from build123d import *

# Parameters (mm, degrees)
F1_DEPTH = 30
F2_R     = 3


with BuildPart() as f1:
    # F0 (on Front) → F1 (new body)
    with BuildSketch(Plane.XZ):
        with BuildLine():
            ThreePointArc((180, -20.182252), (0, -38.788033), (-180, -20.182252))
            Line((-180, -20.182252), (-180, -58.968014))
            ThreePointArc((-180, -58.968014), (0, -76.788032), (180, -58.968014))
            Line((180, -58.968014), (180, -20.182252))
        make_face()
    extrude(amount=-F1_DEPTH)

    # F2
    f2_edges = [f1.edges().sort_by_distance(p)[0] for p in [
        (-180, 15, -20.182252),
        (-180, 15, -58.968014),
        (-180, 0, -39.575133),
        (-180, 30, -39.575133),
        (180, 15, -58.968014),
        (180, 15, -20.182252),
        (180, 0, -39.575133),
        (180, 30, -39.575133),
        (0, 0, -38.788033),
        (0, 30, -38.788033),
        (0, 0, -76.788032),
        (0, 30, -76.788032),
    ]]
    fillet(f2_edges, radius=F2_R)


solid = f1.part
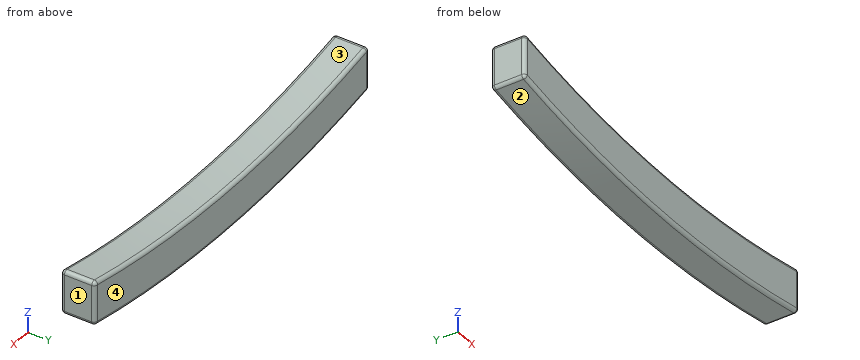
CAD build for the part. Positions are in the model's coordinates, mm. Face numbers are marked on the shaded views. Round coordinates to 2 decimals unless told otherwise and drop trailing zeros. Loops run counter-clockwise (first coordinate to the right, second up) from the corner with the lowest first, then second, coordinate; pieces in that order, holes last. Notation, with made-up numbers: (56.5, -21) - (100.5, -21) arc R24 cw to (100.5, -10) - close; hole circle Ø9 at (-38.75, 35). An arc over 180 degrees is marked (long way). Put each result on its own line as item: value.
1. Wall check: line 1 (Y direction, x = 96, z = -34.5); line 2 (X direction, y = 26.5, z = -59); line 3 (Y direction, x = 59, z = -73). Give the ranges that are in metal, low to high.
Geometry check:
line 1: 0.8 to 29.2
line 2: -178.67 to 178.67
line 3: 0.21 to 29.79
2. Slice it at A-A on y = 19.75. List the corners of the cut face in (x, z).
Geometry check:
outline: (-180, -56.51) arc R3 ccw to (-177.58, -59.45) arc R918 ccw to (177.58, -59.45) arc R3 ccw to (180, -56.51) - (180, -23.87) arc R3 ccw to (176.4, -20.93) arc R880 cw to (-176.4, -20.93) arc R3 ccw to (-180, -23.87) - close
3. Two-plate mould, pull along X, no slides. Class the marked faces 1, 2, 3 and 4: released by +X, released by -X, zero draft, split by the parting line, or undercut.
Geometry check:
face 1: released by +X
face 2: split by the parting line
face 3: undercut
face 4: zero draft
